Could you check a few things on this drawing? It's one solid part, dimensions in mm from its lowest x, y, z. A direction names the side the tool comes from. Give positions to 0.01 mm unless a question says otherwise; leave off trailing zeros. Order: outer loops, then holes, each group sorted by start corner. A loop starts at its lowest first (then second) coordinate and runs counter-clockwise, first axis right, second up. Notation, with made-up numbers: (-15, 22) - (24, 22) arc R22 ccw to (24, 52) - close; hole circle Ø8 at (-26.75, -24.5). An arc over 180 degrees is marked (long way). Return JSON: item names as keys, results as strings.
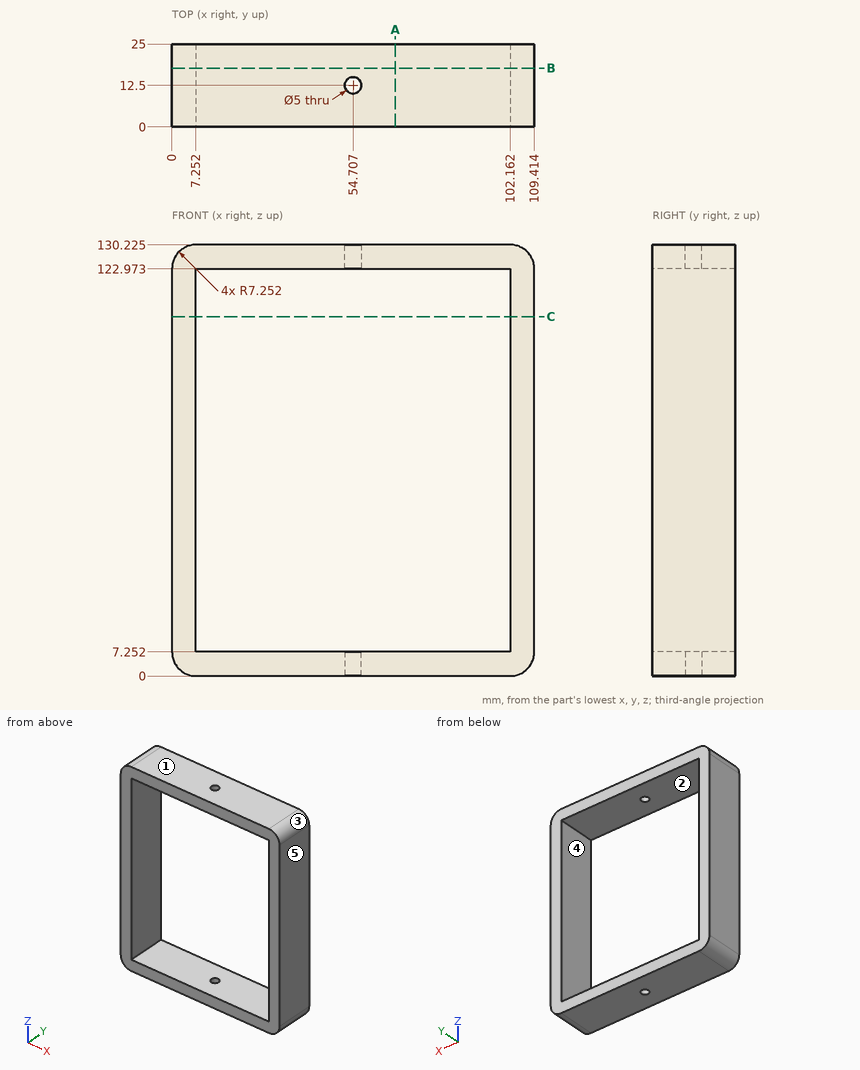
1. On a 3-axis mill with a long thin cutter (end or side, diameter ignored), from which of +Z, -Z, +X, -X, +Y, -Y can I reach the whole of each face in a straight line? I mean the marked faces 4 and 5. Say none if no direction works.
Checks:
{"face 4": "+Y, -Y", "face 5": "+Z, -Z, +X, +Y, -Y"}
2. Suppose I cut it at A-A (x = 67.5). List the corners of the cut face in (y, z) for me (1 decimal).
Checks:
{"outline": "(0, 0) - (25, 0) - (25, 7.3) - (0, 7.3) - close; (0, 123) - (25, 123) - (25, 130.2) - (0, 130.2) - close"}
3. If I drill on L1, parallel to Z at x = 46.5, y = 16 (1 decimal); L2, parallel to X at y = 11.5, z = 77.5 (1 decimal); L3, parallel to X at y = 12.5, z = 5.5 (1 decimal), over which ranges is the centre line in solid material (lowest first)? Write a range as [from, to].
Checks:
{"L1": "[0, 7.3], [123, 130.2]", "L2": "[0, 7.3], [102.2, 109.4]", "L3": "[0.2, 52.2], [57.2, 109.2]"}
4. Thinking about a two-plate mould opening in X: for the marked faces 1, 2 and 3, which applies, +X half, -X half, draft (parallel to the pull), parting line (faces both ways), or undercut?
Checks:
{"face 1": "draft", "face 2": "undercut", "face 3": "+X half"}
5. Suppose I cut it at B-B (y = 17.75). List the corners of the cut face in (x, z) for me (1 decimal), plus the area to 3 significant figures.
Checks:
{"outline": "(0, 7.3) arc R7.3 ccw to (7.3, 0) - (102.2, 0) arc R7.3 ccw to (109.4, 7.3) - (109.4, 123) arc R7.3 ccw to (102.2, 130.2) - (7.3, 130.2) arc R7.3 ccw to (0, 123) - close; hole (7.3, 7.3) - (102.2, 7.3) - (102.2, 123) - (7.3, 123) - close", "area": "3,220 mm^2"}
6. Suppose I cut it at C-C (z = 108.5). List the corners of the cut face in (x, y) for me (1 decimal).
Checks:
{"outline": "(0, 0) - (7.3, 0) - (7.3, 25) - (0, 25) - close; (102.2, 0) - (109.4, 0) - (109.4, 25) - (102.2, 25) - close"}
